from build123d import *

# Parameters (mm, degrees)
SKETCH_W        = 302
SKETCH_H        = 112
PAD_DEPTH       = 6
SKETCH001_W     = 287
SKETCH001_H     = 97
POCKET_DEPTH    = 4
SKETCH002_W     = 302
SKETCH002_H     = 112
SKETCH002_W_2   = 296.96
SKETCH002_H_2   = 106.96
POCKET001_DEPTH = 3.02
FILLET_R        = 3
FILLET001_R     = 5
FILLET002_R     = 5
FILLET003_R     = 3
FILLET004_R     = 2
FILLET005_R     = 2
FILLET006_R     = 5
FILLET007_R     = 3
FILLET008_R     = 2
FILLET009_R     = 5
FILLET010_R     = 3
FILLET011_R     = 2
SKETCH003_W     = 80
SKETCH003_H     = 5
POCKET002_DEPTH = 1.25
SKETCH004_W     = 5
SKETCH004_H     = 32.5
POCKET003_DEPTH = 1.25
FILLET012_R     = 1
FILLET013_R     = 1
FILLET014_R     = 1
FILLET015_R     = 1
FILLET016_R     = 1
FILLET017_R     = 1
FILLET018_R     = 1
FILLET019_R     = 1
FILLET020_R     = 1
FILLET021_R     = 1
FILLET022_R     = 1
FILLET023_R     = 1
FILLET024_R     = 1
FILLET025_R     = 1
FILLET026_R     = 1
FILLET027_R     = 1
FILLET028_R     = 1
FILLET029_R     = 1
FILLET030_R     = 1
FILLET031_R     = 1


with BuildPart() as part:
    # Sketch → Pad (new body)
    with BuildSketch(Plane.XY):
        Rectangle(SKETCH_W, SKETCH_H)
    extrude(amount=PAD_DEPTH)

    # Sketch001 (on Face6 of Pad) → Pocket (cut)
    with BuildSketch(Plane.XY.offset(6)):
        Rectangle(SKETCH001_W, SKETCH001_H)
    extrude(amount=-POCKET_DEPTH, mode=Mode.SUBTRACT)

    # Sketch002 (on Face5 of Pocket) → Pocket001 (cut)
    with BuildSketch(Plane.XY.offset(6)):
        Rectangle(SKETCH002_W, SKETCH002_H)
        Rectangle(SKETCH002_W_2, SKETCH002_H_2, mode=Mode.SUBTRACT)
    extrude(amount=-POCKET001_DEPTH, mode=Mode.SUBTRACT)

    # Fillet
    fillet_edges = [part.edges().sort_by_distance(p)[0] for p in [
        (-148.48, -53.48, 4.49),
    ]]
    fillet(fillet_edges, radius=FILLET_R)

    # Fillet001
    fillet001_edges = [part.edges().sort_by_distance(p)[0] for p in [
        (-151, -56, 1.49),
    ]]
    fillet(fillet001_edges, radius=FILLET001_R)

    # Fillet002
    fillet002_edges = [part.edges().sort_by_distance(p)[0] for p in [
        (-151, 56, 1.49),
    ]]
    fillet(fillet002_edges, radius=FILLET002_R)

    # Fillet003
    fillet003_edges = [part.edges().sort_by_distance(p)[0] for p in [
        (-148.48, 53.48, 4.49),
    ]]
    fillet(fillet003_edges, radius=FILLET003_R)

    # Fillet004
    fillet004_edges = [part.edges().sort_by_distance(p)[0] for p in [
        (-143.5, 48.5, 4),
    ]]
    fillet(fillet004_edges, radius=FILLET004_R)

    # Fillet005
    fillet005_edges = [part.edges().sort_by_distance(p)[0] for p in [
        (-143.5, -48.5, 4),
    ]]
    fillet(fillet005_edges, radius=FILLET005_R)

    # Fillet006
    fillet006_edges = [part.edges().sort_by_distance(p)[0] for p in [
        (151, -56, 1.49),
    ]]
    fillet(fillet006_edges, radius=FILLET006_R)

    # Fillet007
    fillet007_edges = [part.edges().sort_by_distance(p)[0] for p in [
        (148.48, -53.48, 4.49),
    ]]
    fillet(fillet007_edges, radius=FILLET007_R)

    # Fillet008
    fillet008_edges = [part.edges().sort_by_distance(p)[0] for p in [
        (143.5, -48.5, 4),
    ]]
    fillet(fillet008_edges, radius=FILLET008_R)

    # Fillet009
    fillet009_edges = [part.edges().sort_by_distance(p)[0] for p in [
        (151, 56, 1.49),
    ]]
    fillet(fillet009_edges, radius=FILLET009_R)

    # Fillet010
    fillet010_edges = [part.edges().sort_by_distance(p)[0] for p in [
        (148.48, 53.48, 4.49),
    ]]
    fillet(fillet010_edges, radius=FILLET010_R)

    # Fillet011
    fillet011_edges = [part.edges().sort_by_distance(p)[0] for p in [
        (143.5, 48.5, 4),
    ]]
    fillet(fillet011_edges, radius=FILLET011_R)

    # Sketch003 (on Face1 of Fillet011) → Pocket002 (cut)
    with BuildSketch(Plane.XY.offset(6)):
        with Locations((0, 51)):
            Rectangle(SKETCH003_W, SKETCH003_H)
        with Locations((-95, 51)):
            Rectangle(SKETCH003_W, SKETCH003_H)
        with Locations((95, 51)):
            Rectangle(SKETCH003_W, SKETCH003_H)
        with Locations((95, -51)):
            Rectangle(SKETCH003_W, SKETCH003_H)
        with Locations((0, -51)):
            Rectangle(SKETCH003_W, SKETCH003_H)
        with Locations((-95, -51)):
            Rectangle(SKETCH003_W, SKETCH003_H)
    extrude(amount=-POCKET002_DEPTH, mode=Mode.SUBTRACT)

    # Sketch004 (on Face25 of Pocket002) → Pocket003 (cut)
    with BuildSketch(Plane.XY.offset(6)):
        with Locations((-146, 23.75)):
            Rectangle(SKETCH004_W, SKETCH004_H)
        with Locations((-146, -23.75)):
            Rectangle(SKETCH004_W, SKETCH004_H)
        with Locations((146, 23.75)):
            Rectangle(SKETCH004_W, SKETCH004_H)
        with Locations((146, -23.75)):
            Rectangle(SKETCH004_W, SKETCH004_H)
    extrude(amount=-POCKET003_DEPTH, mode=Mode.SUBTRACT)

    # Fillet012
    fillet012_edges = [part.edges().sort_by_distance(p)[0] for p in [
        (-55, 48.5, 5.375),
    ]]
    fillet(fillet012_edges, radius=FILLET012_R)

    # Fillet013
    fillet013_edges = [part.edges().sort_by_distance(p)[0] for p in [
        (-40, 48.5, 5.375),
    ]]
    fillet(fillet013_edges, radius=FILLET013_R)

    # Fillet014
    fillet014_edges = [part.edges().sort_by_distance(p)[0] for p in [
        (-135, 48.5, 5.375),
    ]]
    fillet(fillet014_edges, radius=FILLET014_R)

    # Fillet015
    fillet015_edges = [part.edges().sort_by_distance(p)[0] for p in [
        (-143.5, 40, 5.375),
    ]]
    fillet(fillet015_edges, radius=FILLET015_R)

    # Fillet016
    fillet016_edges = [part.edges().sort_by_distance(p)[0] for p in [
        (-143.5, 7.5, 5.375),
    ]]
    fillet(fillet016_edges, radius=FILLET016_R)

    # Fillet017
    fillet017_edges = [part.edges().sort_by_distance(p)[0] for p in [
        (-143.5, -7.5, 5.375),
    ]]
    fillet(fillet017_edges, radius=FILLET017_R)

    # Fillet018
    fillet018_edges = [part.edges().sort_by_distance(p)[0] for p in [
        (-143.5, -40, 5.375),
    ]]
    fillet(fillet018_edges, radius=FILLET018_R)

    # Fillet019
    fillet019_edges = [part.edges().sort_by_distance(p)[0] for p in [
        (-135, -48.5, 5.375),
    ]]
    fillet(fillet019_edges, radius=FILLET019_R)

    # Fillet020
    fillet020_edges = [part.edges().sort_by_distance(p)[0] for p in [
        (-40, -48.5, 5.375),
    ]]
    fillet(fillet020_edges, radius=FILLET020_R)

    # Fillet021
    fillet021_edges = [part.edges().sort_by_distance(p)[0] for p in [
        (-55, -48.5, 5.375),
    ]]
    fillet(fillet021_edges, radius=FILLET021_R)

    # Fillet022
    fillet022_edges = [part.edges().sort_by_distance(p)[0] for p in [
        (40, -48.5, 5.375),
    ]]
    fillet(fillet022_edges, radius=FILLET022_R)

    # Fillet023
    fillet023_edges = [part.edges().sort_by_distance(p)[0] for p in [
        (55, -48.5, 5.375),
    ]]
    fillet(fillet023_edges, radius=FILLET023_R)

    # Fillet024
    fillet024_edges = [part.edges().sort_by_distance(p)[0] for p in [
        (135, -48.5, 5.375),
    ]]
    fillet(fillet024_edges, radius=FILLET024_R)

    # Fillet025
    fillet025_edges = [part.edges().sort_by_distance(p)[0] for p in [
        (143.5, -40, 5.375),
    ]]
    fillet(fillet025_edges, radius=FILLET025_R)

    # Fillet026
    fillet026_edges = [part.edges().sort_by_distance(p)[0] for p in [
        (143.5, 7.5, 5.375),
    ]]
    fillet(fillet026_edges, radius=FILLET026_R)

    # Fillet027
    fillet027_edges = [part.edges().sort_by_distance(p)[0] for p in [
        (143.5, -7.5, 5.375),
    ]]
    fillet(fillet027_edges, radius=FILLET027_R)

    # Fillet028
    fillet028_edges = [part.edges().sort_by_distance(p)[0] for p in [
        (135, 48.5, 5.375),
    ]]
    fillet(fillet028_edges, radius=FILLET028_R)

    # Fillet029
    fillet029_edges = [part.edges().sort_by_distance(p)[0] for p in [
        (143.5, 40, 5.375),
    ]]
    fillet(fillet029_edges, radius=FILLET029_R)

    # Fillet030
    fillet030_edges = [part.edges().sort_by_distance(p)[0] for p in [
        (55, 48.5, 5.375),
    ]]
    fillet(fillet030_edges, radius=FILLET030_R)

    # Fillet031
    fillet031_edges = [part.edges().sort_by_distance(p)[0] for p in [
        (40, 48.5, 5.375),
    ]]
    fillet(fillet031_edges, radius=FILLET031_R)


solid = part.part
The listing builds one solid part. Answer for the finished solid, in the listing's coordinates (mm). A direction names the side the tool comes from. Round coordinates to 2 decimals unless told otherwise and drop trailing zeros. Order: outer loops, then holes, each group sorted by start corner. A loop starts at its lowest first (then second) coordinate and runs counter-clockwise, first axis right, second up. Notation, with made-up numbers: (-18, 66) - (30, 66) arc R24 ccw to (30, 93) - close; hole circle Ø1 at (57, 87.25). An arc over 180 degrees is marked (long way). Write item = value, one per line. Start each with the question number.
1) Straight lines are drawn through the part: L1, parallel to X at y = -12.5, z = 4.6; L2, parallel to X at y = -1.5, z = 2.35; L3, parallel to Y at x = 1, z = 3.5. For each, find the intervals that lie inside material, in ascending order.
2) Given pin 1 (1.5 mm diameter, centred on x = -7, y = -50, fed in from +Z); pin 2 (4 mm diameter, centred on x = 32, y = 10, fed in from +Z); pin 3 (0.6 mm diameter, centred on y = 51, z = 5, fed in from +X), each flat-ended and moving along its own axis, determine where each tip first touches the part or whether it passes through.
3) Section A-A, the plane x = 95.5 is taken. Write down the section's boundary in (y, z).
4) For a pull along X with two mould halves and no side action, classify faces 1 (the cylindrical face through (-150, 54, 2)), 2 (the flat face through (94, -51, 4.75)), 3 (the flat face through (47, -51, 6)) as released by +X, released by -X, zero draft, split by the parting line, or undercut.
5) For faces 4 (the flat face through (-1, 51, 4.75)), 5 (the flat face through (-146, 0, 6)), determine the directions among +Z, -Z, +X, -X, +Y, -Y from which every point of the face is accessible in a straight line to the end or side of a thin tool.
6) Section B-B, the plane y = 32 is taken. Write down the section's boundary in (x, z), plus the area to 3 significant figures.
Results list:
q1.L1 = -148.48 to -143.5, 143.5 to 148.48
q1.L2 = -151 to -143.5, 143.5 to 151
q1.L3 = -53.48 to -48.5, 48.5 to 53.48
q2.pin_1 = 4.75
q2.pin_2 = 2
q2.pin_3 = 148.47
q3.outline = (-56, 0) - (56, 0) - (56, 2.98) - (53.48, 2.98) - (53.48, 4.75) - (48.5, 4.75) - (48.5, 2) - (-48.5, 2) - (-48.5, 4.75) - (-53.48, 4.75) - (-53.48, 2.98) - (-56, 2.98) - close
q4.face_1 = released by -X
q4.face_2 = undercut
q4.face_3 = zero draft
q5.face_4 = +Z, +Y, -Y
q5.face_5 = +Z, +X, -X, +Y, -Y
q6.outline = (-151, 0) - (151, 0) - (151, 2.98) - (148.48, 2.98) - (148.48, 4.75) - (143.5, 4.75) - (143.5, 2) - (-143.5, 2) - (-143.5, 4.75) - (-148.48, 4.75) - (-148.48, 2.98) - (-151, 2.98) - close
q6.area = 636 mm^2
